Geometry check sheet. Reference: the model listing, model coordinates, mm. Give positions to 0.01 mm unless a question says otherwise; leave off trailing zeros. Order: outer loops, then holes, each group sorted by start corner. A loop starts at its lowest first (then second) coordinate and runs counter-clockwise, first axis right, second up.
from build123d import *

# Parameters (mm, degrees)
F2_DEPTH = 30
F3_R     = 14.99999


# Not quite as in the source:
# - a fillet or chamfer is up to 0.001 mm smaller than in the source, because OpenCascade refuses the exact size


with BuildPart() as f2:
    # F1 (on offset) → F2 (new body)
    with BuildSketch(Plane.XY.offset(750)):
        Polygon((640, 0), (-640, 0), (-640, -80), (-780, -80), (-780, -480), (-480, -550), (480, -550), (780, -480), (780, -80), (640, -80), align=None)
    extrude(amount=F2_DEPTH)

    # F3 (radius 15 in the source; OpenCascade refuses exactly that, so slightly less here)
    f3_edges = [f2.edges().sort_by_distance(p)[0] for p in [
        (-630, -515, 780),
        (-780, -480, 765),
        (-480, -550, 765),
        (-630, -515, 750),
        (480, -550, 765),
        (0, -550, 750),
        (0, -550, 780),
        (780, -480, 765),
        (630, -515, 750),
        (630, -515, 780),
    ]]
    fillet(f3_edges, radius=F3_R)


solid = f2.part
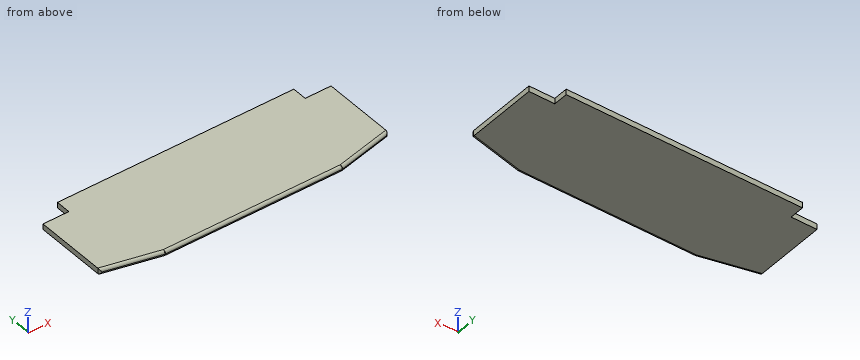
Item 1: Gauge pin test, flat ends, axial feed: pin 1 (9 mm diameter, centred on y = -49.5, z = 757.5, fed in from +X); pin 2 (15 mm diameter, centred on y = -20, z = 762.5, fed in from -X); pin 3 (4 mm diameter, centred on x = 442, z = 774.5, fed in from -Y). Record the tip position at first contact, or that the pin passes through.
Reported:
pin 1: stops at x = 640
pin 2: stops at x = -640
pin 3: stops at y = -547.99
Item 2: Sectioned sample at A-A (z = 771.25). Enter the section's corners in (x, y), and give its area (3 significant figures).
Reported:
outline: (-780, -468.1) arc R15 ccw to (-774.18, -479.96) - (-481.37, -548.28) arc R13.64 ccw to (-478.27, -548.64) - (478.27, -548.64) arc R13.64 ccw to (481.37, -548.28) - (774.18, -479.96) arc R15 ccw to (780, -468.1) - (780, -80) - (640, -80) - (640, 0) - (-640, 0) - (-640, -80) - (-780, -80) - close
area: 812,000 mm2
Item 3: Scan lines: L1, parallel to Y at x = -33, z = 762.75; L2, parallel to Y at x = 343.5, z = 764; L3, parallel to X at y = -41.5, z = 757.25. Record each from-to range of solid material in increasing order.
Reported:
L1: y = -549.83 to 0
L2: y = -549.97 to 0
L3: x = -640 to 640
